Autodesk Inventor part; units mm, degrees
ref_plane "YZ Plane" through (0, 0, 0) normal (1, 0, 0) x (0, 1, 0)
ref_plane "XZ Plane" through (0, 0, 0) normal (0, 1, 0) x (-1, 0, 0)
ref_plane "XY Plane" through (0, 0, 0) normal (0, 0, 1) x (1, 0, 0)
sketch "Sketch1" plane through (0, 0, 0) normal (0, 1, 0) x (-1, 0, 0)
  line L0 (0, 0) -> (50, 0)
  line L1 (50, 0) -> (50, -50)
  line L2 (50, -50) -> (0, -50)
  line L3 (0, -50) -> (0, 0)
  dimension "d0" = 50
  dimension "d1" = 50
extrude "Extrusion1" add sketch "Sketch1" along normal blind 900
sketch "Sketch2" plane through (0, 900, 0) normal (0, 1, 0) x (1, 0, 0)
  line L0 (0, 50) -> (-50, 50)
  line L1 (-50, 50) -> (-50, 0)
  line L2 (-50, 0) -> (0, 0)
  line L3 (0, 0) -> (0, 50)
  line L4 (-47.5, 2.5) -> (-2.5, 2.5)
  line L5 (-2.5, 2.5) -> (-2.5, 47.5)
  line L6 (-2.5, 47.5) -> (-47.5, 47.5)
  line L7 (-47.5, 47.5) -> (-47.5, 2.5)
  line L8 (-47.5, 2.5) -> (-2.5, 47.5) construction
  line L9 (-2.5, 2.5) -> (-47.5, 47.5) construction
  point P0 (-25, 25)
  dimension "d4" = 45
  dimension "d5" = 45
extrude "Extrusion2" cut sketch "Sketch2" against normal up to surface (900 mm away) contours L7 L6 L5 L4
properties part number "metalonmeio"
Source: CAD feature listing. Evaluate the final solid. Frame: model axes, mm. A direction names the side the tool comes from. Round coordinates to 2 decimals unless told otherwise and drop trailing zeros. Loops run counter-clockwise (first coordinate to the right, second up) from the corner with the lowest first, then second, coordinate; pieces in that order, holes last. Notation, with made-up numbers: (76, 24) - (123, 24) arc R22 cw to (123, 33) - close; hole circle Ø7 at (-32, -21). An arc over 180 degrees is marked (long way). Write item = value, one per line. Start each with the question number.
(1) Ray query, line 1 along X through (y, z) = (538, -4). Return the intervals inside material, ascending. Write a range as from..to.
(2) Set-up query: faces 5 (the face through (-25, 456, -47.5)), 6 (the face through (-23, 900, -49)). Return all of +Z, -Z, +X, -X, +Y, -Y with unobstructed straight access to the full face (end or side cutting, diameter ignored); none if empty.
(3) Section query A-A, the plane z = -17.5. Output: boundary loops of the cut face in (x, y).
(4) Section query B-B, the plane x = -19. Output: boundary loops of the cut face in (y, z), plus the area to 3 significant figures.
(5) Section query C-C, the plane y = 180. Output: boundary loops of the cut face in (x, z), plus the area to 3 significant figures.
(6) Pull-direction query (X, two-part tool) for faces 1 (the face through (0, 444, -25)), 2 (the face through (-2.5, 456, -25)), 3 (the face through (-50, 444, -25)), 4 (the face through (-25, 444, 0)); classes: +X half, -X half, draft (parallel to the pull), parting line (faces both ways), or undercut.
Conclusion:
q1.line_1 = -50..-47.5, -2.5..0
q2.face_5 = +Y, -Y
q2.face_6 = +Z, -Z, +X, -X, +Y
q3.outline = (-50, 0) - (-47.5, 0) - (-47.5, 900) - (-50, 900) - close; (-2.5, 0) - (0, 0) - (0, 900) - (-2.5, 900) - close
q4.outline = (0, -50) - (900, -50) - (900, -47.5) - (0, -47.5) - close; (0, -2.5) - (900, -2.5) - (900, 0) - (0, 0) - close
q4.area = 4,500 mm2
q5.outline = (-50, -50) - (0, -50) - (0, 0) - (-50, 0) - close; hole (-47.5, -47.5) - (-2.5, -47.5) - (-2.5, -2.5) - (-47.5, -2.5) - close
q5.area = 475 mm2
q6.face_1 = +X half
q6.face_2 = undercut
q6.face_3 = -X half
q6.face_4 = draft
